Geometry check sheet. Reference: the model listing, model coordinates, mm. A direction names the side the tool comes from. Round coordinates to 2 decimals unless told otherwise and drop trailing zeros. Write each loop counter-clockwise with the first axis right and the second up, starting at its lowest first coordinate (ties: lowest second). Pieces come first, ordered by that corner, then holes. Notation, with made-up numbers: M 9,34 L 13,34 A10 ccw 13,47 Z; hole C 4,86.5 d1. An arc over 180 degrees is marked long. Put each result on its own line as item: value. Start each with the question number.
(1) Section check A-A on y = 128.5. Count the separate pieces of the cut face and the enclosed holes in it, then the cut area to 3 significant figures.
(2) Gauge pin test, flat ends, axial feed: pin 1 (8 mm diameter, centred on x = 55.5, z = 90, fed in from +Y); pin 2 (3 mm diameter, centred on x = 31.5, z = 101, fed in from +Y). Record the tip position at first contact, or that the pin passes through.
(3) Tool access check on faces 3 (the cylindrical face through (100.19, 58.7, -109.84)), 4 (the flat face through (-3, 0, -2)). Record the directions out of +Z, -Z, +X, -X, +Y, -Y that give a thin tool (end or side, any length) a straight path to the whole face; none if there is none.
(4) Section check C-C on x = 149. Record the cut outline in (y, z).
(5) Section check B-B on z = 0. Record the cut outline in (x, y), then the cut area to 3 significant figures.
(6) Material ranges on probe 1 along X at (y, z) = (60, -99); probe 2 along Z at (x, y) = (-147, 74.5); probe 3 along X at (y, z) = (68, 0), recorded low to high.
(7) Mould release check, pull along Z, two halves, no side actions. Record for faces 1 (the flat face through (-3, 143, -2)), 2 (the cylindrical face through (-34.99, 125.74, -144.63)): pulls with the +Z half, pulls with the -Z half, needs draft (parallel to the pull), parting line crosses it, or undercut.
from build123d import *

# Parameters (mm, degrees)
SKETCH_1_W          = 438
SKETCH_1_H          = 338
EXTRUDE_1_DEPTH     = 143
SKETCH_2_R          = 50
CUT_EXTRUDE_1_DEPTH = 135
SKETCH_4_R          = 57.5
CUT_EXTRUDE_2_DEPTH = 35


with BuildPart() as part:
    # Эскиз1 → Бобышка-Вытянуть1 (new body)
    with BuildSketch(Plane(origin=(0, 0, 0), x_dir=(1, 0, 0), z_dir=(0, 1, 0))):
        Rectangle(SKETCH_1_W, SKETCH_1_H)
    extrude(amount=EXTRUDE_1_DEPTH)

    # Эскиз2 → Вырез-Вытянуть1 (cut)
    with BuildSketch(Plane(origin=(0, 143, 0), x_dir=(1, 0, 0), z_dir=(0, 1, 0))):
        with Locations(Location((-149, 99, 0), (0, 0, 270))):
            Circle(SKETCH_2_R)
        with Locations(Location((0, 99, 0), (0, 0, 270))):
            Circle(SKETCH_2_R)
        with Locations(Location((0, -99, 0), (0, 0, 270))):
            Circle(SKETCH_2_R)
        with Locations(Location((-149, -99, 0), (0, 0, 270))):
            Circle(SKETCH_2_R)
        with Locations(Location((-74.5, 0, 0), (0, 0, 270))):
            Circle(SKETCH_2_R)
        with Locations(Location((149, 99, 0), (0, 0, 270))):
            Circle(SKETCH_2_R)
        with Locations(Location((149, -99, 0), (0, 0, 270))):
            Circle(SKETCH_2_R)
        with Locations(Location((74.5, 0, 0), (0, 0, 270))):
            Circle(SKETCH_2_R)
    extrude(amount=-CUT_EXTRUDE_1_DEPTH, mode=Mode.SUBTRACT)

    # Эскиз4 → Вырез-Вытянуть2 (cut)
    with BuildSketch(Plane(origin=(0, 143, 0), x_dir=(1, 0, 0), z_dir=(0, 1, 0))):
        with Locations(Location((-149, 99, 0), (0, 0, 270))):
            Circle(SKETCH_4_R)
        with Locations(Location((0, 99, 0), (0, 0, 270))):
            Circle(SKETCH_4_R)
        with Locations(Location((0, -99, 0), (0, 0, 270))):
            Circle(SKETCH_4_R)
        with Locations(Location((-149, -99, 0), (0, 0, 270))):
            Circle(SKETCH_4_R)
        with Locations(Location((-74.5, 0, 0), (0, 0, 270))):
            Circle(SKETCH_4_R)
        with Locations(Location((149, 99, 0), (0, 0, 270))):
            Circle(SKETCH_4_R)
        with Locations(Location((149, -99, 0), (0, 0, 270))):
            Circle(SKETCH_4_R)
        with Locations(Location((74.5, 0, 0), (0, 0, 270))):
            Circle(SKETCH_4_R)
    extrude(amount=-CUT_EXTRUDE_2_DEPTH, mode=Mode.SUBTRACT)


solid = part.part
Answers follow:
1. separate pieces: 1
1. enclosed holes: 8
1. area: 64,900 mm^2
2. pin 1: stops at y = 143
2. pin 2: stops at y = 8
3. face 3: +Y
3. face 4: +Z, -Z, +X, -X, -Y
4. outline: M 0,-169 L 143,-169 L 143,-156.5 L 108,-156.5 L 108,-149 L 8,-149 L 8,-49 L 108,-49 L 108,-41.5 L 143,-41.5 L 143,41.5 L 108,41.5 L 108,49 L 8,49 L 8,149 L 108,149 L 108,156.5 L 143,156.5 L 143,169 L 0,169 Z
5. outline: M -219,0 L 219,0 L 219,143 L 132,143 L 132,108 L 124.5,108 L 124.5,8 L 24.5,8 L 24.5,108 L 17,108 L 17,143 L -17,143 L -17,108 L -24.5,108 L -24.5,8 L -124.5,8 L -124.5,108 L -132,108 L -132,143 L -219,143 Z
5. area: 34,600 mm^2
6. probe 1: x = -219 to -199, -99 to -50, 50 to 99, 199 to 219
6. probe 2: z = -169 to -148.96, -49.04 to 49.04, 148.96 to 169
6. probe 3: x = -219 to -124.5, -24.5 to 24.5, 124.5 to 219
7. face 1: needs draft
7. face 2: undercut
